Autodesk Inventor part; units mm, degrees
ref_plane "YZ Plane" through (0, 0, 0) normal (1, 0, 0) x (0, 1, 0)
ref_plane "XZ Plane" through (0, 0, 0) normal (0, 1, 0) x (-1, 0, 0)
ref_plane "XY Plane" through (0, 0, 0) normal (0, 0, 1) x (1, 0, 0)
sketch "Boceto1" plane through (0, 0, 0) normal (0, 0, 1) x (1, 0, 0)
  line L0 (78.56, -21.6086) -> (46.5862, 76.7964)
  line L1 (82.0867, -22.7545) -> (78.56, -21.6086)
  line L2 (82.0867, -22.7545) -> (48.7659, 79.7964)
  line L3 (46.5862, 76.7964) -> (48.7659, 79.7964)
  line L4 (-5.1483, -82.4262) -> (78.56, -21.6086)
  line L5 (-5.1483, -86.1344) -> (-5.1483, -82.4262)
  line L6 (-5.1483, -86.1344) -> (82.0867, -22.7545)
  line L7 (78.56, -21.6086) -> (82.0867, -22.7545)
  line L8 (-88.8566, -21.6086) -> (-5.1483, -82.4262)
  line L9 (-88.8566, -21.6086) -> (-92.3834, -22.7545)
  line L10 (-5.1483, -86.1344) -> (-92.3834, -22.7545)
  line L11 (-5.1483, -86.1344) -> (-5.1483, -82.4262)
  line L12 (-56.8829, 76.7964) -> (-88.8566, -21.6086)
  line L13 (-59.0626, 79.7964) -> (-56.8829, 76.7964)
  line L14 (-59.0626, 79.7964) -> (-92.3834, -22.7545)
  line L15 (-88.8566, -21.6086) -> (-92.3834, -22.7545)
  line L16 (46.5862, 76.7964) -> (-56.8829, 76.7964)
  line L17 (48.7659, 79.7964) -> (46.5862, 76.7964)
  line L18 (48.7659, 79.7964) -> (-59.0626, 79.7964)
  line L19 (-56.8829, 76.7964) -> (-59.0626, 79.7964)
  circle A0 centre (-5.1483, 5.5899) radius 71.2065
  line L20 (-92.3834, -22.7545) -> (-59.0626, 79.7964)
  line L21 (-59.0626, 79.7964) -> (48.7659, 79.7964)
  line L22 (48.7659, 79.7964) -> (82.0867, -22.7545)
  line L23 (82.0867, -22.7545) -> (-5.1483, -86.1344)
  line L24 (-5.1483, -86.1344) -> (-92.3834, -22.7545)
  line L25 (-5.1483, -85.5164) -> (81.4989, -22.5635)
  line L26 (81.4989, -22.5635) -> (48.4026, 79.2964)
  line L27 (48.4026, 79.2964) -> (-58.6993, 79.2964)
  line L28 (-58.6993, 79.2964) -> (-91.7956, -22.5635)
  line L29 (-91.7956, -22.5635) -> (-5.1483, -85.5164)
  point P0 (0, 0)
  point P1 (-5.1483, 5.5899)
  dimension "d0" = 0.5
extrude "Extrusión1" add sketch "Boceto1" along normal blind 1.2
properties part number "Pentagono"
For this review, take the finished solid that the model builds, in its own axes (mm). Coordinates: 2 decimals unless noted, no trailing zeros. Loops run counter-clockwise (first coordinate to the right, second up) from the corner with the lowest first, then second, coordinate; pieces in that order, holes last.
1. Add section C-C, the plane x = -46. Give the boundary of the cut face in (y, z).
2. Add section B-B, the plane y = 22. Give the boundary of the cut face in (x, z), then the cut area to 3 significant figures.
3. Add section A-A, the plane z = 0.5. Give the boundary of the cut face in (x, y).
4. For line 1 (Y direction, x = -3, z = 0.5); line 2 (Y direction, x = -32, z = 0.45); line 3 (X direction, y = 56.5, z = 0.3), list the stretches that pass through material, from the lowest coordinate up.
Result:
1. outline: (-56.45, 0) - (79.8, 0) - (79.8, 1.2) - (-56.45, 1.2) - close
2. outline: (-77.84, 0) - (67.55, 0) - (67.55, 1.2) - (-77.84, 1.2) - close
2. area: 174 mm2
3. outline: (-92.38, -22.75) - (-5.15, -86.13) - (82.09, -22.75) - (48.77, 79.8) - (-59.06, 79.8) - close
4. line 1: y = -84.57 to 79.8
4. line 2: y = -66.63 to 79.8
4. line 3: x = -66.63 to 56.34
